The listing builds one solid part. Answer for the finished solid, in the listing's coordinates (mm). A direction names the side the tool comes from. Coordinates: 2 decimals unless noted, no trailing zeros. Order: outer loops, then holes, each group sorted by start corner. A loop starts at its lowest first (then second) coordinate and runs counter-clockwise, first axis right, second up. Notation, with made-up numbers: M -32.75,88.5 L -19.75,88.5 A22 cw -19.75,126.5 Z; hole C 49,-32.5 d6. An arc over 180 degrees is marked long. One line per item, written item: value. Start each with the question number.
Q1. Straight lines are drawn through the part: line 1 along Z through (x, y) = (-28.35, 0); line 2 along Z through (x, y) = (-24.25, 0); line 3 along Z through (x, y) = (-19.5, -0.05). For each, find the intervals that lie inside material, in ascending order. Write a range as [from, to].
Q2. Determine the mould class of faces 4 (the flat face through (18.4, -2, -1)), 5 (the conical face through (-22.91, 0.04, 0.13)), 6 (the cylindrical face through (30.36, -0.27, 1.22)) for opening direction Z: pulls with the +Z half, pulls with the -Z half, needs draft (parallel to the pull), parting line crosses it, or undercut.
Q3. The part is cut by section A-A on x = 27. Give the vertices of the cut face in (y, z).
Q4. This flat-tipped pin is pushed along its axis until it touches: pin 1 Ø1.1 at (y, z) = (0, 0) entering from -X. Where does it stop, or does it pass through?
Q5. For faces 1 (the flat face through (32.9, 0, 0)), 2 (the cylindrical face through (24, -1.5, -0.07)), 3 (the cylindrical face through (-25.272, -0.235, 0.747)), determine the directions among +Z, -Z, +X, -X, +Y, -Y from which every point of the face is accessible in a straight line to the end or side of a thin tool.
Q6. The part is cut by section B-B on x = -5. Give the vertices of the cut face in (y, z).
Autodesk Inventor part; units mm, degrees
ref_plane "YZ Plane" through (0, 0, 0) normal (1, 0, 0) x (0, 1, 0)
ref_plane "XZ Plane" through (0, 0, 0) normal (0, 1, 0) x (-1, 0, 0)
ref_plane "XY Plane" through (0, 0, 0) normal (0, 0, 1) x (1, 0, 0)
sketch "Sketch1" plane through (0, 0, 0) normal (0, 0, 1) x (1, 0, 0)
  line L0 (-18.4, 0) -> (18.4, 0)
  line L1 (18.4, 0) -> (18.4, 2.45)
  line L2 (18.4, 2.45) -> (-18.4, 2.45)
  line L3 (-18.4, 2.45) -> (-18.4, 0)
  line L4 (-18.4, 0) -> (-19.9, 0)
  line L5 (-19.9, 0) -> (-19.9, 1.95)
  line L6 (-19.9, 1.95) -> (-18.4, 1.95)
  line L7 (-18.4, 1.95) -> (-18.4, 0)
  line L8 (-19.9, 0) -> (-29.3, 0)
  line L9 (-29.3, 0) -> (-29.3, 1.6)
  line L10 (-29.3, 1.6) -> (-19.9, 1.6)
  line L11 (-19.9, 1.6) -> (-19.9, 0)
  line L12 (18.4, 0) -> (20.2, 0)
  line L13 (20.2, 0) -> (20.2, 1.95)
  line L14 (20.2, 1.95) -> (18.4, 1.95)
  line L15 (18.4, 1.95) -> (18.4, 0)
  line L16 (20.2, 0) -> (27.9, 0)
  line L17 (27.9, 0) -> (27.9, 1.5)
  line L18 (27.9, 1.5) -> (20.2, 1.5)
  line L19 (20.2, 1.5) -> (20.2, 0)
  line L20 (27.9, 0) -> (32.9, 0)
  line L21 (32.9, 0) -> (32.9, 1.25)
  line L22 (32.9, 1.25) -> (27.9, 1.25)
  line L23 (27.9, 1.25) -> (27.9, 0)
  point P0 (0, 0)
  point P1 (0, 0)
  dimension "d0" = 9.4
  dimension "d1" = 10.9
  dimension "d2" = 47.7
  dimension "d3" = 3.2
  dimension "d4" = 3.9
  dimension "d5" = 4.9
  dimension "d6" = 3
  dimension "d7" = 49.5
  dimension "d21" = 2.5
  dimension "d22" = 62.2
  dimension "d23" = 5
revolve "Revolution1" add sketch "Sketch1" angle 360 about axis through (-18.4, 0, 0) along (1, 0, 0)
thread "Thread1"
hole "Hole1" at (-29.3, 0, 0) direction (1, 0, 0) diameter 1.567 depth 6 tip angle 118 counterbore diameter 1.9 counterbore depth 2
properties part number "401-05" material "Aluminum-6061"
Output:
1. line 1: z = [-1.6, -0.95], [0.95, 1.6]
1. line 2: z = [-1.6, -0.78], [0.78, 1.6]
1. line 3: z = [-1.95, 1.95]
2. face 4: needs draft
2. face 5: undercut
2. face 6: parting line crosses it
3. outline: C 0,0 d3
4. pin 1: stops at x = -23.16
5. face 1: +Z, -Z, +X, +Y, -Y
5. face 2: +X
5. face 3: -X
6. outline: C 0,0 d4.9
